For this review, take the finished solid that the model builds, in its own axes (mm). A direction names the side the tool comes from. Round coordinates to 2 decimals unless told otherwise and drop trailing zeros. Write each loop counter-clockwise with the first axis right and the second up, starting at its lowest first coordinate (ties: lowest second). Pieces come first, ordered by that corner, then holes. Notation, with made-up numbers: M 48.5,-38.5 L 88.5,-38.5 A13 cw 88.5,-18.5 Z; hole C 83.5,-16.5 d3. An arc over 180 degrees is marked long. Use one line per item in the form item = value. Start each with the question number.
Item 1: For line 1 (Y direction, x = 2.75, z = 0); line 2 (Y direction, x = 2, z = 0); line 3 (Z direction, x = 1, y = 36.75), list the stretches that pass through material, from the lowest coordinate up. Write a range as [from, to].
Item 2: Add section C-C (z = 2). State the section outline as (x, y) points, and give its area (3 significant figures).
Item 3: Draft analysis for pull direction Y (two halves, no side actions). For faces 1 (the cylindrical face through (0.07, 37.68, -0.59)), 2 (the flat face through (0, 10, -1.05)), 3 (the cylindrical face through (0.07, 39.07, 3.5)), state which applies: released by +Y, released by -Y, zero draft, split by the parting line, or undercut.
Item 4: For faces 4 (the flat face through (0, 9, 1.05)), 5 (the cylindrical face through (0, 2.5, 1.5)), 6 (the flat face through (0, 0, 2)), list the 3-axis set-ups (+Z, -Z, +X, -X, +Y, -Y) from which the entire face can be reached by the end or side of a thin tool; tool diameter is ignored.
Item 5: Add section B-B (y = 36.75). State the section outline as (x, z) points.
Item 6: For P1, Ø1.8, axis at y = 36.75, z = 0, coming from the -X side; P2, Ø3, axis at x = -1.5, y = 23, coming from the -Z side; P3, Ø2, axis at y = 5.5, z = -1, coming from the +X side; P4, Ø1.3, axis at x = 1, y = 5.5, coming from the +Z side, all flat-tipped, find the tip position at first contact; note any pin that passes through.
Autodesk Inventor part; units mm, degrees
ref_plane "YZ Plane" through (0, 0, 0) normal (1, 0, 0) x (0, 1, 0)
ref_plane "XZ Plane" through (0, 0, 0) normal (0, 1, 0) x (-1, 0, 0)
ref_plane "XY Plane" through (0, 0, 0) normal (0, 0, 1) x (1, 0, 0)
sketch "Sketch1" plane through (0, 0, 0) normal (0, 1, 0) x (-1, 0, 0)
  circle A0 centre (0, 0) radius 2.4
  dimension "d0" = 4.8
extrude "Extrusion1" add sketch "Sketch1" along normal blind 33
sketch "Sketch2" plane through (0, 33, 0) normal (0, 1, 0) x (1, 0, 0)
  line L0 (-5, 0) -> (5, 0)
  line L1 (-5, 0) -> (-5, -5)
  line L2 (-5, -5) -> (5, -5)
  line L3 (5, -5) -> (5, 0)
  line L4 (-5, 0) -> (-5, 5)
  line L5 (-5, 5) -> (5, 5)
  line L6 (5, 5) -> (5, 0)
  point P0 (0, 0)
  dimension "d4" = 10
  dimension "d5" = 5
  dimension "d6" = 5
extrude "Extrusion2" add sketch "Sketch2" along normal blind 7.5
fillet "Fillet1" radius 5 2 edges at (0, 40.5, 5) (0, 40.5, -5)
sketch "Sketch3" plane through (5, 33, 5) normal (1, 0, 0) x (0, 0, -1)
  line L0 (10, 0) -> (0, 0)
  line L1 (5, 0) -> (5, 7.5)
  arc A0 (10, 2.5) -> (0, 2.5) centre (5, 2.5) ccw
  line L2 (5, 0) -> (5, 3.75)
  circle A1 centre (5, 3.75) radius 1.1
  point P0 (5, -33)
  dimension "d10" = 2.2
extrude "Extrusion3" cut sketch "Sketch3" against normal through all
sketch "Sketch5" plane through (0, 0, 0) normal (0, -1, 0) x (1, 0, 0)
  circle A0 centre (0, 0) radius 2.4
  circle A1 centre (0, 0) radius 1.5
  dimension "d19" = 3
extrude "Extrusion5" cut sketch "Sketch5" against normal blind 5 contours A1
sketch "Sketch6" plane through (5, 33, 5) normal (1, 0, 0) x (0, 0, -1)
  line L0 (5, -33) -> (5, -32)
  line L1 (5, -32) -> (5, -24)
  line L2 (5, -24) -> (5, -32) construction
  line L3 (3.95, -25.05) -> (3.95, -30.95)
  line L4 (6.05, -30.95) -> (6.05, -25.05)
  arc A0 (6.05, -25.05) -> (3.95, -25.05) centre (5, -25.05) ccw
  arc A1 (3.95, -30.95) -> (6.05, -30.95) centre (5, -30.95) ccw
  line L5 (5, -33) -> (5, -24) construction
  line L6 (7.4, -33) -> (2.6, -33)
  line L7 (3.95, -31.95) -> (3.95, -25.05)
  line L8 (6.05, -25.05) -> (6.05, -31.95)
  arc A2 (3.95, -31.95) -> (6.05, -31.95) centre (5, -31.95) ccw
  arc A3 (6.05, -25.05) -> (3.95, -25.05) centre (5, -25.05) ccw
  line L9 (3.95, -31.95) -> (3.95, -33)
  line L10 (6.05, -31.95) -> (6.05, -33)
  line L11 (3.95, -33) -> (6.05, -33)
  line L12 (5, -24) -> (5, 0)
  line L13 (7.4, 0) -> (2.6, 0)
  line L14 (5, 0) -> (5, -33)
  line L15 (5, -16.5) -> (7.4, -16.5)
  line L16 (7.4, -33) -> (7.4, 0)
  line L17 (5, -16.5) -> (5, -28) construction
  line L18 (3.95, -17.55) -> (3.95, -26.95)
  line L19 (6.05, -26.95) -> (6.05, -17.55)
  arc A4 (6.05, -17.55) -> (3.95, -17.55) centre (5, -17.55) ccw
  arc A5 (3.95, -26.95) -> (6.05, -26.95) centre (5, -26.95) ccw
  point P0 (5, -28.5)
  point P1 (6.05, -30.95)
  point P2 (5, -22.25)
  dimension "d22" = 1
  dimension "d23" = 8
  dimension "d24" = 2.1
extrude "Extrusion6" cut sketch "Sketch6" against normal through all contours A2 L7 A1 L0 | A2 L10 L6 | L6 L9 A2 | L0 A1 L8 A2 | A1 L3 A5 L1 | L1 A5 L4 A1 | A5 L3 A0 L1 | L1 A0 L4 A5 | L12 A4 L19 A0 | A0 L18 A4 L12
properties part number "pist"
Calculated:
q1.line_1 = [33, 35.65], [37.85, 40.5]
q1.line_2 = [16.5, 35.65], [37.85, 40.5]
q1.line_3 = [-4.84, -1.1], [1.1, 4.84]
q2.outline = M -5,33 L -1.33,33 L -1.33,0 L 1.33,0 L 1.33,33 L 5,33 L 5,40.08 L -5,40.08 Z
q2.area = 158 mm^2
q3.face_1 = undercut
q3.face_2 = zero draft
q3.face_3 = released by +Y
q4.face_4 = +X, -X, -Y
q4.face_5 = -Y
q4.face_6 = +Z, -Z, +X, -X, -Y
q5.outline = M -5,-4.84 L 5,-4.84 L 5,-1.1 L -5,-1.1 Z; M -5,1.1 L 5,1.1 L 5,4.84 L -5,4.84 Z
q6.P1 = through
q6.P2 = -2.4
q6.P3 = 2.16
q6.P4 = 2.37
